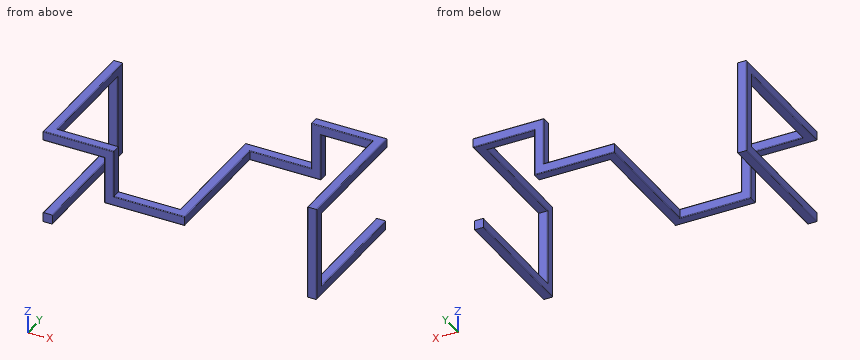
from build123d import *

# Parameters (mm, degrees)
F0_W      = 40
F0_H      = 40
F1_DEPTH  = 560
F2_W      = 40
F2_H      = 40
F3_DEPTH  = 360
F4_W      = 40
F4_H      = 40
F5_DEPTH  = 520
F6_W      = 40
F6_H      = 40
F7_DEPTH  = 260
F8_W      = 40
F8_H      = 40
F9_DEPTH  = 200
F10_W     = 40
F10_H     = 40
F11_DEPTH = 300
F12_W     = 40
F12_H     = 40
F13_DEPTH = 520
F14_W     = 40
F14_H     = 40
F15_DEPTH = 300
F16_W     = 40
F16_H     = 40
F17_DEPTH = 200
F18_W     = 40
F18_H     = 40
F19_DEPTH = 260
F20_W     = 40
F20_H     = 40
F21_DEPTH = 520
F22_W     = 40
F22_H     = 40
F23_DEPTH = 360
F24_W     = 40
F24_H     = 40
F25_DEPTH = 510
F26_R     = 3


with BuildPart() as f1:
    # F0 (on Front) → F1 (new body)
    with BuildSketch(Plane.XZ):
        with Locations((20, 20)):
            Rectangle(F0_W, F0_H)
    extrude(amount=-F1_DEPTH)

    # F2 (on face) → F3 (join)
    with BuildSketch(Plane.XY.offset(40)):
        with Locations((20, 540)):
            Rectangle(F2_W, F2_H)
    extrude(amount=F3_DEPTH)

    # F4 (on face) → F5 (join)
    with BuildSketch(Plane.XZ.offset(-520)):
        with Locations((20, 380)):
            Rectangle(F4_W, F4_H)
    extrude(amount=F5_DEPTH)

    # F6 (on face) → F7 (join)
    with BuildSketch(Plane.YZ.offset(40)):
        with Locations((20, 380)):
            Rectangle(F6_W, F6_H)
    extrude(amount=F7_DEPTH)

    # F8 (on face) → F9 (join)
    with BuildSketch(Plane(origin=(0, 0, 360), x_dir=(1, 0, 0), z_dir=(0, 0, -1))):
        with Locations((280, -20)):
            Rectangle(F8_W, F8_H)
    extrude(amount=F9_DEPTH)

    # F10 (on face) → F11 (join)
    with BuildSketch(Plane.YZ.offset(300)):
        with Locations((20, 180)):
            Rectangle(F10_W, F10_H)
    extrude(amount=F11_DEPTH)

    # F12 (on face) → F13 (join)
    with BuildSketch(Plane(origin=(0, 40, 0), x_dir=(-1, 0, 0), z_dir=(0, 1, 0))):
        with Locations((-580, 180)):
            Rectangle(F12_W, F12_H)
    extrude(amount=F13_DEPTH)

    # F14 (on face) → F15 (join)
    with BuildSketch(Plane.YZ.offset(600)):
        with Locations((540, 180)):
            Rectangle(F14_W, F14_H)
    extrude(amount=F15_DEPTH)

    # F16 (on face) → F17 (join)
    with BuildSketch(Plane.XY.offset(200)):
        with Locations((880, 540)):
            Rectangle(F16_W, F16_H)
    extrude(amount=F17_DEPTH)

    # F18 (on face) → F19 (join)
    with BuildSketch(Plane.YZ.offset(900)):
        with Locations((540, 380)):
            Rectangle(F18_W, F18_H)
    extrude(amount=F19_DEPTH)

    # F20 (on face) → F21 (join)
    with BuildSketch(Plane.XZ.offset(-520)):
        with Locations((1140, 380)):
            Rectangle(F20_W, F20_H)
    extrude(amount=F21_DEPTH)

    # F22 (on face) → F23 (join)
    with BuildSketch(Plane(origin=(0, 0, 360), x_dir=(1, 0, 0), z_dir=(0, 0, -1))):
        with Locations((1140, -20)):
            Rectangle(F22_W, F22_H)
    extrude(amount=F23_DEPTH)

    # F24 (on face) → F25 (join)
    with BuildSketch(Plane(origin=(0, 40, 0), x_dir=(-1, 0, 0), z_dir=(0, 1, 0))):
        with Locations((-1140, 20)):
            Rectangle(F24_W, F24_H)
    extrude(amount=F25_DEPTH)

    # F26
    f26_edges = [f1.edges().sort_by_distance(p)[0] for p in [
        (0, 280, 400),
        (150, 0, 400),
        (170, 40, 400),
        (40, 300, 400),
        (0, 260, 40),
        (130, 0, 360),
        (260, 0, 260),
        (300, 0, 300),
        (430, 40, 200),
        (450, 0, 200),
        (430, 0, 160),
        (40, 520, 200),
        (0, 560, 200),
        (0, 280, 0),
        (40, 260, 40),
        (560, 300, 200),
        (600, 260, 200),
        (710, 560, 200),
        (730, 520, 200),
        (750, 520, 160),
        (560, 300, 160),
        (1120, 275, 0),
        (1160, 295, 40),
        (1120, 295, 40),
        (1120, 40, 200),
        (1160, 0, 200),
        (1120, 0, 200),
        (1120, 280, 360),
        (1160, 280, 400),
        (1120, 260, 400),
        (1010, 560, 400),
        (990, 520, 400),
        (1010, 520, 360),
        (900, 520, 260),
        (860, 520, 300),
        (860, 560, 300),
        (1160, 300, 360),
        (1160, 275, 0),
        (1030, 560, 360),
        (730, 560, 160),
        (900, 560, 260),
        (600, 260, 160),
        (410, 40, 160),
        (150, 40, 360),
        (300, 40, 300),
        (1160, 40, 200),
        (40, 560, 200),
        (40, 280, 0),
        (0, 520, 200),
        (0, 260, 360),
        (40, 280, 360),
        (260, 40, 260),
    ]]
    fillet(f26_edges, radius=F26_R)


solid = f1.part
Model file for the job. Use its own axes, mm. Give positions to 0.01 mm unless a question says otherwise; leave off trailing zeros. Order: outer loops, then holes, each group sorted by start corner. A loop starts at its lowest first (then second) coordinate and runs counter-clockwise, first axis right, second up. Notation, with made-up numbers: M 68.5,58 L 75.5,58 A23 cw 75.5,88 Z; hole C 1.5,36 d2. An arc over 180 degrees is marked long. Write item = value, one per line.
Q1. Flat gauge pins, fed straight in: pin 1 (20 mm diameter, centred on x = 1131, z = 29.5, fed in from +Y); pin 2 (17 mm diameter, centred on x = 14.5, z = 170.5, fed in from -Y); pin 3 (8 mm diameter, centred on x = 685.5, z = 162, fed in from +Y). Where does each tip first touch, or does it go through?
Derived:
pin_1 = 550
pin_2 = 520
pin_3 = 560
Q2. Cut at C-C, the plane x = 703. List the corners of the cut face in (y, z).
Derived:
outline = M 520,163 A3 ccw 523,160 L 557,160 A3 ccw 560,163 L 560,197 A3 ccw 557,200 L 523,200 A3 ccw 520,197 Z
Q3. Cut at A-A, the plane z = 68.5. List the corners of the cut face in (x, y).
Derived:
outline = M 0,523 A3 ccw 3,520 L 37,520 A3 ccw 40,523 L 40,557 A3 ccw 37,560 L 3,560 A3 ccw 0,557 Z; M 1120,3 A3 ccw 1123,0 L 1157,0 A3 ccw 1160,3 L 1160,37 A3 ccw 1157,40 L 1123,40 A3 ccw 1120,37 Z
Q4. Drill centre lines: line 1 (X direction, y = 501.5, z = 38); line 2 (Z direction, x = 478.5, y = 23); line 3 (Y direction, x = 545, z = 199.5). Where is each one in solid material? Low to high. Write a range as [from, to].
Derived:
line_1 = [0.17, 39.83], [1120.17, 1159.83]
line_2 = [160, 200]
line_3 = [1.34, 38.66]
Q5. Cut at B-B, the plane z = 290. Count the separate pieces of the cut face and the enclosed holes in it, then the cut area to 3 significant figures.
Derived:
separate_pieces = 4
enclosed_holes = 0
area = 6,370 mm2
